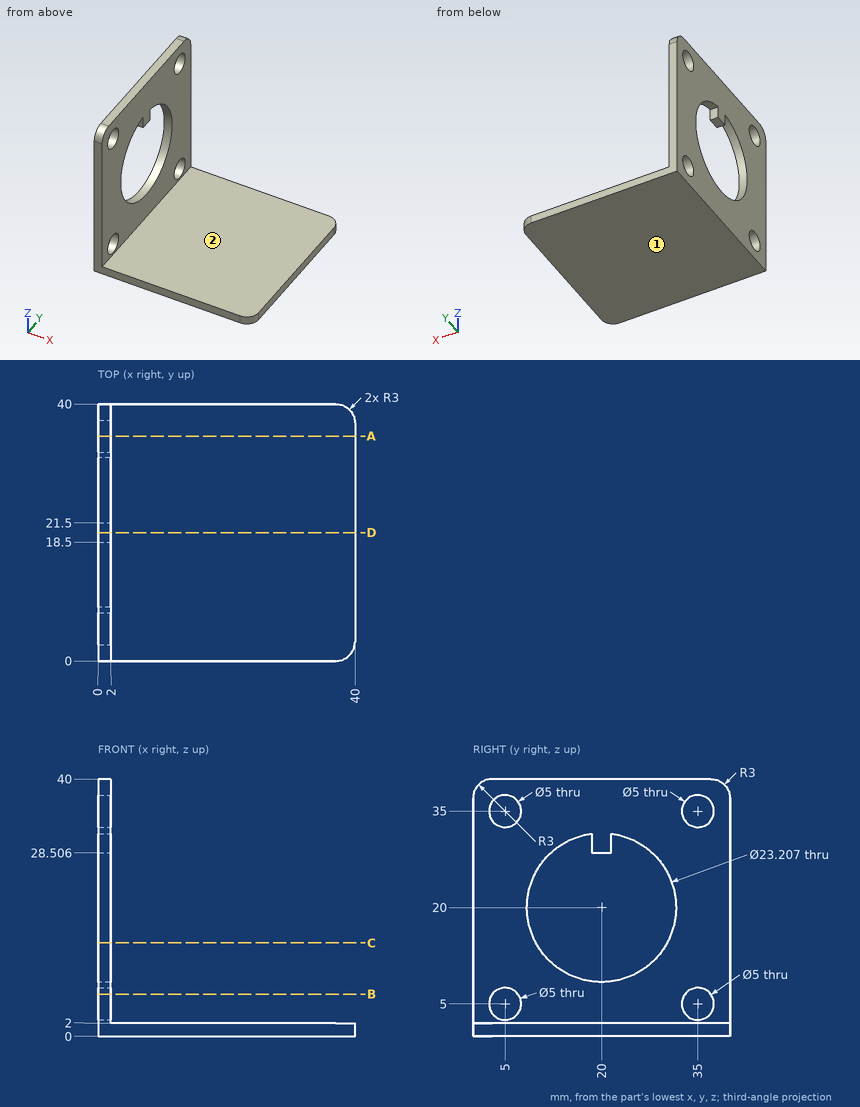
Verification items for this drawing (mm, ordinates from the low corner). A direction names the side the tool comes from. Coordinates: 2 decimals unless noted, no trailing zeros. Write each loop counter-clockwise with the first axis right and the second up, starting at its lowest first coordinate (ties: lowest second). Pieces come first, ordered by that corner, then holes. Notation, with made-up numbers: (-28.75, 52) -> (9.25, 52) arc R19 ccw to (9.25, 62) -> close; hole circle Ø5 at (87, -19). An arc over 180 degrees is marked (long way). Use CSV: the item, a comma, the result in double quotes. Start each with the question number.
Item 1: Depth check by flat-ended pin: pin 1 Ø3 at (y, z) = (35, 5) entering from +X; pin 2 Ø19 at (y, z) = (21, 16.5) entering from +X; pin 3 Ø8 at (x, y) = (26, 23.5) entering from +Z. Enter the tip coordinate at first touch or a pass-through.
Item 2: Cross-section at B-B, the plane z = 6.5. Record the cut outline in (x, y).
Item 3: Cross-section at C-C, the plane z = 14.5. Record the cut outline in (x, y), plus the area to 3 significant figures.
Item 4: Thickness scan on line 1 (Z direction, x = 1, y = 5); line 2 (Z direction, x = 1, y = 20); line 3 (X direction, y = 23, z = 35.5). Record the ranges inside material, lowest first.
Item 5: Set-up check for the marked faces 1 and 2: record each of +Z, -Z, +X, -X, +Y, -Y from which the full face is reachable in a straight line by a thin tool's end or side.
Item 6: Cross-section at D-D, the plane y = 20. Record the cut outline in (x, z), plus the area to 3 significant figures.
Item 7: Cross-section at A-A, the plane y = 35. Record the cut outline in (x, z).
Answers:
1,pin 1,"through"
1,pin 2,"x = 2"
1,pin 3,"z = 2"
2,outline,"(0, 0) -> (2, 0) -> (2, 3) -> (0, 3) -> close; (0, 7) -> (2, 7) -> (2, 33) -> (0, 33) -> close; (0, 37) -> (2, 37) -> (2, 40) -> (0, 40) -> close"
3,outline,"(0, 0) -> (2, 0) -> (2, 9.78) -> (0, 9.78) -> close; (0, 30.22) -> (2, 30.22) -> (2, 40) -> (0, 40) -> close"
3,area,"39.1 mm^2"
4,line 1,"0 to 2.5, 7.5 to 32.5, 37.5 to 40"
4,line 2,"0 to 8.4, 28.51 to 40"
4,line 3,"0 to 2"
5,face 1,"-Z, +X, -X, +Y, -Y"
5,face 2,"+Z, +X, +Y, -Y"
6,outline,"(0, 0) -> (40, 0) -> (40, 2) -> (2, 2) -> (2, 8.4) -> (0, 8.4) -> close; (0, 28.51) -> (2, 28.51) -> (2, 40) -> (0, 40) -> close"
6,area,"116 mm^2"
7,outline,"(0, 0) -> (40, 0) -> (40, 2) -> (2, 2) -> (2, 2.5) -> (0, 2.5) -> close; (0, 7.5) -> (2, 7.5) -> (2, 32.5) -> (0, 32.5) -> close; (0, 37.5) -> (2, 37.5) -> (2, 40) -> (0, 40) -> close"
